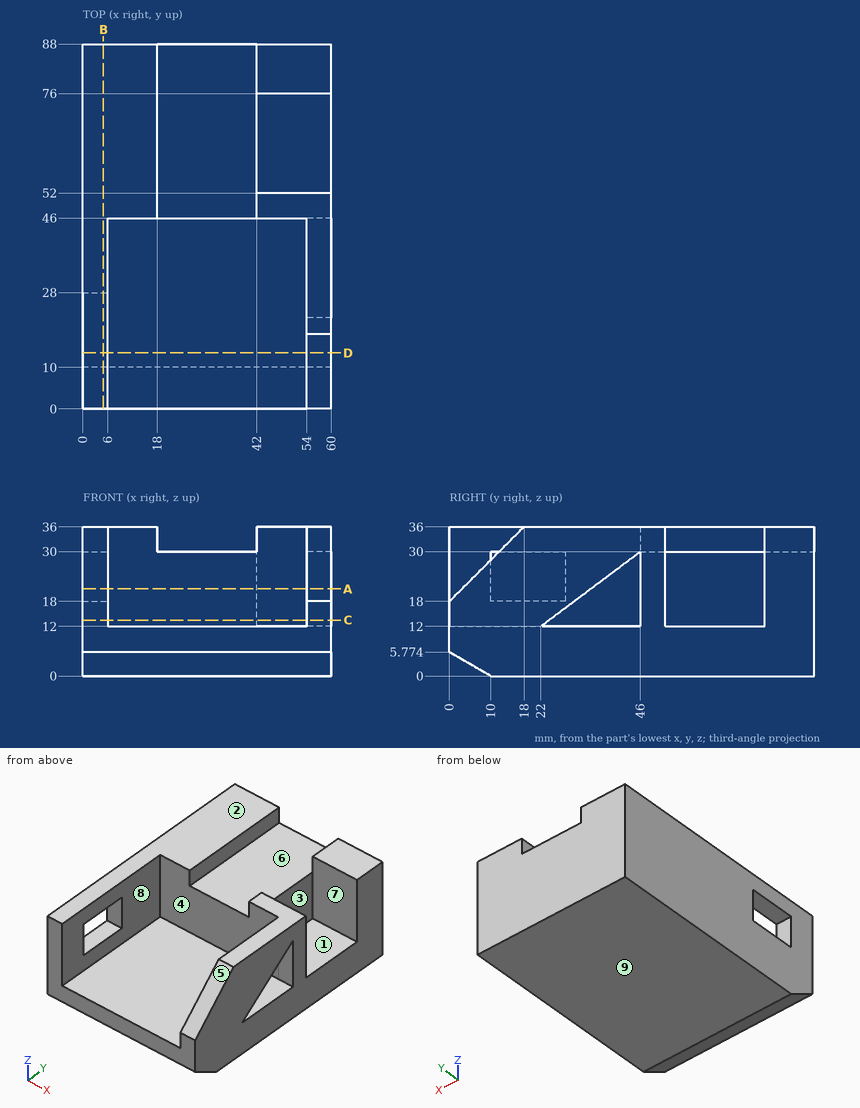
The figure shows three views and two pictorial views of one solid part (mm, origin at its lowest corner). Answer the questions. A direction names the side the tool comes from. Give positions to 0.01 mm unless a question says otherwise; leave off trailing zeros. Write each loop counter-clockwise with the first axis right and the second up, starting at its lowest first coordinate (ties: lowest second). Pieces come first, ordered by that corner, then holes. Notation, with made-up numbers: M 88,82 L 121,82 A27 cw 121,116 Z; hole C 11,-32 d6. An arc over 180 degrees is marked long. Write each question's results on one line, items separated by ' | '.
Q1. For a pull along Y with two mould halves and no side action, classify the marked faces 1, 2, 3 and 4 as released by +Y, released by -Y, zero draft, split by the parting line, or undercut.
Output values:
face 1: undercut | face 2: zero draft | face 3: undercut | face 4: released by -Y
Q2. Section B-B, the plane x = 5 is taken. Write down the section's boundary in (y, z), then the cut area to 3 significant figures.
Output values:
outline: M 0,5.77 L 10,0 L 88,0 L 88,36 L 0,36 Z; hole M 10,18 L 28,18 L 28,30 L 10,30 Z | area: 2,920 mm2
Q3. Section A-A, the plane z = 21 is taken. Write down the section's boundary in (x, y).
Output values:
outline: M 0,0 L 6,0 L 6,10 L 0,10 Z; M 0,28 L 6,28 L 6,46 L 60,46 L 60,52 L 42,52 L 42,76 L 60,76 L 60,88 L 0,88 Z; M 54,3 L 60,3 L 60,34 L 54,34 Z
Q4. Section C-C, the plane z = 13.5 is taken. Write down the section's boundary in (x, y).
Output values:
outline: M 0,0 L 6,0 L 6,46 L 60,46 L 60,52 L 42,52 L 42,76 L 60,76 L 60,88 L 0,88 Z; M 54,0 L 60,0 L 60,24 L 54,24 Z
Q5. Consider L1, parallel to X at y = 6, z = 23.5; L2, parallel to Y at x = 50, z = 27; L3, parallel to Y at x = 56, z = 24. Determine where each line is inside the solid, lowest interval first. Write a range as from..to.
Output values:
L1: 0..6, 54..60 | L2: 46..52, 76..88 | L3: 6..38, 46..52, 76..88
Q6. Flat-ended cylindrical pins translate along their axes: P1, Ø9, axis at x = 55.5, y = 63, coming from the +Z side; P2, Ø5, axis at x = 58, z = 23.5, coming from the -Y side; P3, Ø12, axis at x = 32, y = 62.5, coming from the +Z side. Find the tip coordinate at first contact, or state that the pin passes through.
Output values:
P1: z = 12 | P2: y = 3 | P3: z = 30
Q7. Section D-D, the plane y = 13.5 is taken. Write down the section's boundary in (x, z).
Output values:
outline: M 0,0 L 60,0 L 60,31.5 L 54,31.5 L 54,12 L 6,12 L 6,18 L 0,18 Z; M 0,30 L 6,30 L 6,36 L 0,36 Z
Q8. A tool of negligible diameter and unlimited length cuts with its end or side. For the marked faces 5, 6, 7, 8 and 9, from which of +Z, -Z, +X, -X, +Y, -Y can it reach the whole face along a straight path? Write none if from no direction.
Output values:
face 5: +Z, +X, -Y | face 6: +Z, +Y, -Y | face 7: +Z, +X | face 8: +Z, -Y | face 9: -Z, +X, -X, +Y, -Y
